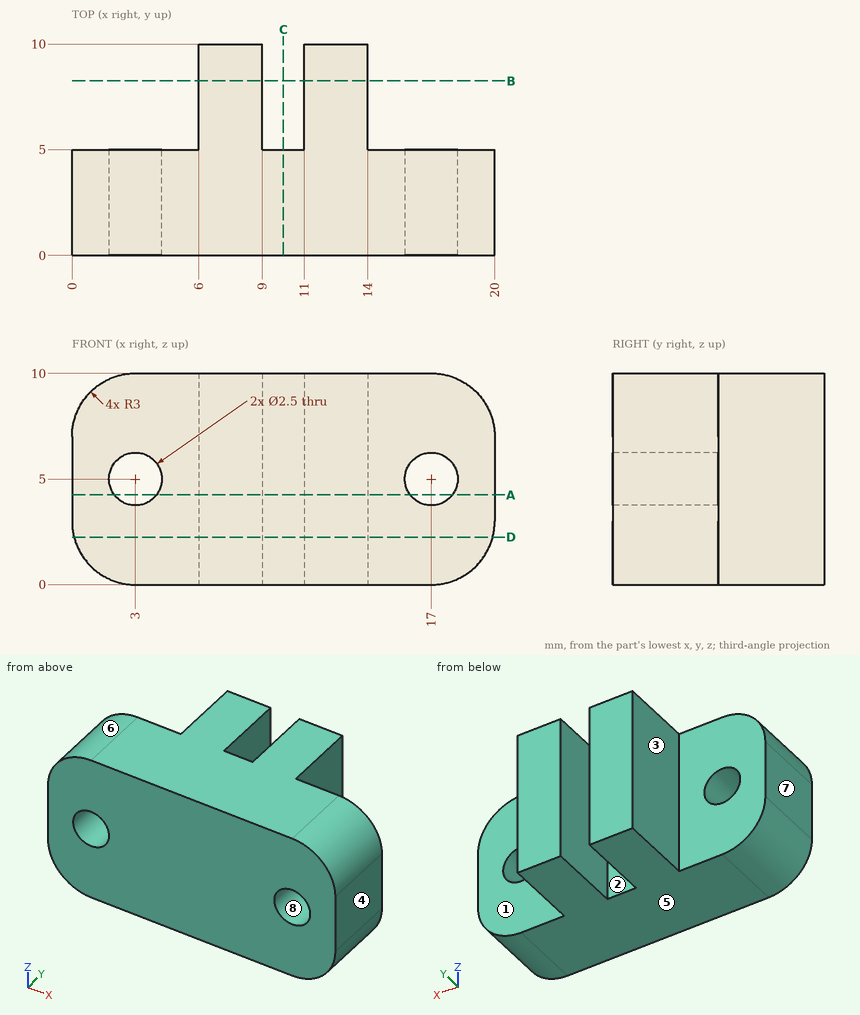
Job drawing, mm, ordinate dimensions from the low corner. One solid piece. A direction names the side the tool comes from. Coordinates: 2 decimals unless noted, no trailing zeros. Write each loop counter-clockwise with the first axis right and the second up, starting at its lowest first coordinate (ties: lowest second). Pieces come first, ordered by that corner, then holes. Notation, with made-up numbers: (-34.75, 40.25) -> (8.25, 40.25) arc R18 cw to (8.25, 69.25) -> close; hole circle Ø3 at (10, 72). An arc over 180 degrees is marked (long way). Use CSV: the item, a comma, the result in double quotes. Start each with the question number.
Item 1: Band-saw the part on C-C, the plane x = 10. Write the cut outline in (y, z), plus the area to 3 significant figures.
Item 2: Two-plate mould, pull along Z, no slides. Class the marked faces 5, 6, 7 and 8: +Z half, -Z half, draft (parallel to the pull), parting line (faces both ways), or undercut.
Item 3: Band-saw the part on B-B, the plane y = 8.25. Write the cut outline in (x, z), plus the area to 3 significant figures.
Item 4: Tool access for the marked faces 1, 2, 3 and 4: list every direction of +Z, -Z, +X, -X, +Y, -Y with a clear straight run to the whole face (end or side of a thin tool).
Item 5: Wall check: probe 1 along Z at (x, y) = (17, 3.8); probe 2 along X at (y, z) = (4.5, 5); probe 3 along X at (y, z) = (7.5, 6). Give the ranges that are in metal, low to high.
Item 6: Band-saw the part on A-A, the plane z = 4.25. Write the cut outline in (x, y).
Item 7: Band-saw the part on D-D, the plane z = 2.25. Write the cut outline in (x, y).
Item 8: Drop flat-ended pins along their axis: P1, Ø3, axis at x = 1.5, z = 5, coming from the +Y side; P2, Ø1, axis at y = 7.5, z = 7, coming from the -X side; P3, Ø1.5, axis at y = 6.5, z = 6.5, coming from the +X side. Give the stop position or say it passes through.
Response values:
1,outline,"(0, 0) -> (5, 0) -> (5, 10) -> (0, 10) -> close"
1,area,"50.0 mm2"
2,face 5,"-Z half"
2,face 6,"+Z half"
2,face 7,"draft"
2,face 8,"undercut"
3,outline,"(6, 0) -> (9, 0) -> (9, 10) -> (6, 10) -> close; (11, 0) -> (14, 0) -> (14, 10) -> (11, 10) -> close"
3,area,"60.0 mm2"
4,face 1,"+Z, -Z, +X, +Y"
4,face 2,"+Z, -Z, +Y"
4,face 3,"+Z, -Z, -X, +Y"
4,face 4,"+Z, -Z, +X, +Y, -Y"
5,probe 1,"z = 0 to 3.75, 6.25 to 10"
5,probe 2,"x = 0 to 1.75, 4.25 to 15.75, 18.25 to 20"
5,probe 3,"x = 6 to 9, 11 to 14"
6,outline,"(0, 0) -> (2, 0) -> (2, 5) -> (0, 5) -> close; (4, 0) -> (16, 0) -> (16, 5) -> (14, 5) -> (14, 10) -> (11, 10) -> (11, 5) -> (9, 5) -> (9, 10) -> (6, 10) -> (6, 5) -> (4, 5) -> close; (18, 0) -> (20, 0) -> (20, 5) -> (18, 5) -> close"
7,outline,"(0.1, 0) -> (19.9, 0) -> (19.9, 5) -> (14, 5) -> (14, 10) -> (11, 10) -> (11, 5) -> (9, 5) -> (9, 10) -> (6, 10) -> (6, 5) -> (0.1, 5) -> close"
8,P1,"stops at y = 5"
8,P2,"stops at x = 6"
8,P3,"stops at x = 14"
